Check sheet for the modelled part. Datum: model origin and axes. Units: mm. A direction names the side the tool comes from. Coordinates: 2 decimals unless noted, no trailing zeros. Write each loop counter-clockwise with the first axis right and the second up, starting at its lowest first coordinate (ties: lowest second). Pieces come first, ordered by that corner, then holes. Notation, with made-up numbers: M 47,-34 L 86,-34 A19 ccw 86,-11 Z; hole C 57,-38.5 d4. An arc over 180 degrees is marked long. Answer as CSV lines item,"result". Start each with the question number.
Q1. Sectioned sample at B-B, the plane z = 11.5. Record the cut outline in (x, y).
Q2. Depth check by flat-ended pin: pin 1 Ø3.5 at (y, z) = (3, 9) entering from -X; pin 2 Ø2.5 at (x, y) = (18, -3) entering from +Z; pin 3 Ø6 at (y, z) = (1, 6) entering from +X. Enter the tip coordinate at first touch or a pass-through.
Q3. Thickness scan on line 1 along Z through (x, y) = (-9, 1); line 2 along X through (y, z) = (2, 9); line 3 along Z through (x, y) = (-13, -0.75). Record the ranges inside material, lowest first. Write a range as from..to.
Q4. Sectioned sample at A-A, the plane y = 4. Record the cut outline in (x, z).
Q5. Sectioned sample at C-C, the plane x = 15.5. Record the cut outline in (y, z), then the cut area to 3 significant figures.
Q6. Access from +Z, -Z, +X, -X, +Y, -Y to the whole of each face (thin tool, end or side, straight path). Record for faces 1 (the flat face through (11, 0, 26)), 2 (the flat face through (17, 0, 20)), 3 (the cylindrical face through (-2.03, -1.11, 33.28)), 4 (the flat face through (-17, 0, 22)).
Q7. Sectioned sample at D-D, the plane y = 0. Record the cut outline in (x, z).
from build123d import *

# Parameters (mm, degrees)
F0_W     = 14.8
F0_H     = 12
F1_DEPTH = 26
F2_W     = 12
F2_H     = 2
F3_DEPTH = 5.2
F5_W     = 17.6
F5_H     = 12
F6_DEPTH = 5.6
F7_R     = 2.895
F8_DEPTH = 3.4


with BuildPart() as f1:
    # F0 (on Top) → F1 (new body)
    with BuildSketch(Plane.XY):
        with Locations((7.4, 0)):
            Rectangle(F0_W, F0_H)
    extrude(amount=F1_DEPTH)

    # F2 (on face) → F3 (join)
    with BuildSketch(Plane.YZ.offset(14.8)):
        with Locations((0, 21)):
            Rectangle(F2_W, F2_H)
    extrude(amount=F3_DEPTH)

    # F4: F1 across plane


with BuildPart() as f1_1:
    add(f1.part)
    add(f1.part.mirror(Plane.YZ))

    # F5 (on face) → F6 (join)
    with BuildSketch(Plane.XY.offset(26)):
        with Locations((-2.2, 0)):
            Rectangle(F5_W, F5_H)
    extrude(amount=F6_DEPTH)

    # F7 (on face) → F8 (join)
    with BuildSketch(Plane.XY.offset(31.6)):
        with Locations((-4.705, 0)):
            Circle(F7_R)
    extrude(amount=F8_DEPTH)


solid = f1_1.part
Output:
1,outline,"M -14.8,-6 L 14.8,-6 L 14.8,6 L -14.8,6 Z"
2,pin 1,"stops at x = -14.8"
2,pin 2,"stops at z = 22"
2,pin 3,"stops at x = 14.8"
3,line 1,"z = 0..31.6"
3,line 2,"x = -14.8..14.8"
3,line 3,"z = 0..26"
4,outline,"M -20,20 L -14.8,20 L -14.8,0 L 14.8,0 L 14.8,20 L 20,20 L 20,22 L 14.8,22 L 14.8,26 L 6.6,26 L 6.6,31.6 L -11,31.6 L -11,26 L -14.8,26 L -14.8,22 L -20,22 Z"
5,outline,"M -6,20 L 6,20 L 6,22 L -6,22 Z"
5,area,"24.0 mm^2"
6,face 1,"+Z, +X, +Y, -Y"
6,face 2,"-Z, +X, +Y, -Y"
6,face 3,"+Z"
6,face 4,"+Z, -X, +Y, -Y"
7,outline,"M -20,20 L -14.8,20 L -14.8,0 L 14.8,0 L 14.8,20 L 20,20 L 20,22 L 14.8,22 L 14.8,26 L 6.6,26 L 6.6,31.6 L -1.81,31.6 L -1.81,35 L -7.6,35 L -7.6,31.6 L -11,31.6 L -11,26 L -14.8,26 L -14.8,22 L -20,22 Z"
